```python
from build123d import *

# Parameters (mm, degrees)
F0_R     = 110.5
F0_R_2   = 95.5
F1_DEPTH = 15
F2_R     = 110
F2_R_2   = 100
F3_DEPTH = 5
F4_R     = 4.15
F5_DEPTH = 25
F6_R     = 6.5
F7_DEPTH = 10


with BuildPart() as f1:
    # F0 (on Top) → F1 (new body)
    with BuildSketch(Plane.XY):
        Circle(F0_R)
        Circle(F0_R_2, mode=Mode.SUBTRACT)
    extrude(amount=F1_DEPTH)

    # F2 (on face) → F3 (cut)
    with BuildSketch(Plane.XY.offset(15)):
        Circle(F2_R)
        Circle(F2_R_2, mode=Mode.SUBTRACT)
    extrude(amount=-F3_DEPTH, mode=Mode.SUBTRACT)

    # F4 (on face) → F5 (cut)
    with BuildSketch(Plane(origin=(0, 0, 0), x_dir=(1, 0, 0), z_dir=(0, 0, -1))):
        with Locations((-74.2462, 74.246224)):
            Circle(F4_R)
        with Locations((-74.2462, -74.246176)):
            Circle(F4_R)
        with Locations((74.2462, 74.246224)):
            Circle(F4_R)
        with Locations((74.2462, -74.246176)):
            Circle(F4_R)
    extrude(amount=-F5_DEPTH, mode=Mode.SUBTRACT)

    # F6 (on face) → F7 (cut)
    with BuildSketch(Plane.XY.offset(15)):
        with Locations((-74.2462, 74.246176)):
            Circle(F6_R)
        with Locations((74.2462, 74.246176)):
            Circle(F6_R)
        with Locations((74.2462, -74.246224)):
            Circle(F6_R)
        with Locations((-74.2462, -74.246224)):
            Circle(F6_R)
    extrude(amount=-F7_DEPTH, mode=Mode.SUBTRACT)


solid = f1.part
```
Source: CAD feature listing. Evaluate the final solid. Frame: model axes, mm. A direction names the side the tool comes from. Round coordinates to 2 decimals unless told otherwise and drop trailing zeros. Loops run counter-clockwise (first coordinate to the right, second up) from the corner with the lowest first, then second, coordinate; pieces in that order, holes last.
1. Contact query for flat-ended pins moving along their axis: pin 1 (1.5 mm diameter, centred on y = -51.5, z = 4, fed in from -X); pin 2 (2 mm diameter, centred on y = -76.5, z = 8.5, fed in from -X); pin 3 (5 mm diameter, centred on x = -33.5, z = 11.5, fed in from -Y); pin 4 (7.5 mm diameter, centred on x = -74.25, y = -74.25, fed in from -Z). Output: stop coordinate, or through.
2. Section query A-A on y = 0. Output: boundary loops of the cut face in (x, z).
3. Access query for faces 1 (the cylindrical face through (78.08, -72.66, 2.46)), 2 (the flat face through (101, 0, 10)). Directions: +Z, -Z, +X, -X, +Y, -Y. A direction counts if a zero-diameter tool reaches every point of the face in a straight line with its end or side. Return the directions, or none.
4. Ray query, L1, parallel to Y at x = -26.5, z = 11; L2, parallel to Y at x = -29, z = 12.75; L3, parallel to X at y = -69, z = 10.25. Return the intervals inside material, ascending.
Answers below:
1. pin 1: stops at x = -98.16
1. pin 2: stops at x = -80.68
1. pin 3: stops at y = -106.06
1. pin 4: passes through
2. outline: (-110.5, 0) - (-95.5, 0) - (-95.5, 15) - (-100, 15) - (-100, 10) - (-110, 10) - (-110, 15) - (-110.5, 15) - close; (95.5, 0) - (110.5, 0) - (110.5, 15) - (110, 15) - (110, 10) - (100, 10) - (100, 15) - (95.5, 15) - close
3. face 1: +Z, -Z
3. face 2: +Z
4. L1: y = -107.28 to -106.76, -96.42 to -91.75, 91.75 to 96.42, 106.76 to 107.28
4. L2: y = -106.63 to -106.11, -95.7 to -90.99, 90.99 to 95.7, 106.11 to 106.63
4. L3: x = -86.31 to -85.67, -70.41 to -66.02, 66.02 to 70.41, 85.67 to 86.31
